Can you work these out from the model? Positions are in its coordinate system, mm. A direction names the side the tool comes from. Give positions to 0.01 mm unless a question says otherwise; leave off trailing zeros. Order: outer loops, then holes, each group sorted by start corner. A loop starts at its lowest first (then second) coordinate and runs counter-clockwise, first axis right, second up.
Item 1: I want a section at C-C, the plane x = 2.5. Write out the boundary of the cut face in (y, z), then the cut area to 3 significant figures.
Item 2: I want a section at A-A, the plane y = 0.2. Write out the boundary of the cut face in (x, z).
Item 3: If I drill on line 1 along Y through (x, z) = (1.25, 1); line 2 along Z through (x, y) = (-0.75, 0.3); line 3 along Z through (x, y) = (-1, 1), over which ranges is the centre line in solid material (lowest first)?
Item 4: If we mould it in two halves opening along Z, with no side actions, what happens to faces 6 (the flat face through (-1.73, 0.74, 4.57)), 7 (the flat face through (-2.957, 1, 5)), 8 (the flat face through (-0.35, 0.74, 0.97))? For each: +Z half, -Z half, draft (parallel to the pull), parting line (faces both ways), or undercut.
Item 5: I want a section at B-B, the plane z = 5. Write out the boundary of the cut face in (x, y), then the cut area to 3 significant figures.
Item 6: I want a section at D-D, the plane z = 2. Write out the boundary of the cut face in (x, y).
Item 7: Which directions (+Z, -Z, +X, -X, +Y, -Y) give clear straight access to the entire face, cutting with the end or side of a thin tool? Please do faces 1 (the flat face through (2.25, 1, -2)), 2 (the flat face through (-0.539, 1, 3)), 3 (the flat face through (-0.324, 1, -3)), 4 (the flat face through (-3.024, 1, 2)), 5 (the flat face through (-1.765, 0.74, 3.095)).
```python
from build123d import *

# Parameters (mm, degrees)
EXTRUDE_1_DEPTH   = 1.5
EXTRUDE_1_2_DEPTH = 1.5
EXTRUDE_1_3_DEPTH = 1.5
SKETCH_2_W        = 6.224573854
SKETCH_2_H        = 11.35798735
EXTRUDE_2_DEPTH   = 0.3


with BuildPart() as part:
    # Sketch 1 → Extrude 1 (new body)
    with BuildSketch(Plane(origin=(0, 0, 0), x_dir=(1, 0, 0), z_dir=(0, 1, 0))):
        Polygon((2.250249032, 2.455487133), (2.250249032, 0.954155558), (-3.02390068, -2.945886183), (-3.02390068, -1.444554608), align=None)
    extrude(amount=EXTRUDE_1_DEPTH)



with BuildPart() as body_2:
    # Sketch 1 → Extrude 1 2 (new body)
    with BuildSketch(Plane(origin=(0, 0, 0), x_dir=(1, 0, 0), z_dir=(0, 1, 0))):
        Polygon((2.093564175, 5.11615287), (2.093564175, 3.614821296), (-0.323874137, 1.827213654), (-0.323874137, 3.328545229), align=None)
    extrude(amount=EXTRUDE_1_2_DEPTH)


with BuildPart() as body_3:
    # Sketch 1 → Extrude 1 3 (new body)
    with BuildSketch(Plane(origin=(0, 0, 0), x_dir=(1, 0, 0), z_dir=(0, 1, 0))):
        Polygon((-0.539241249, -2.188970073), (-0.539241249, -3.690301647), (-2.956679561, -5.477909289), (-2.956679561, -3.976577714), align=None)
    extrude(amount=EXTRUDE_1_3_DEPTH)


with BuildPart() as part_1:
    add(part.part)

    add(body_2.part)  # Extrude 2 merges body 2

    add(body_3.part)  # Extrude 2 merges body 3
    # Sketch 2 → Extrude 2 (add)
    with BuildSketch(Plane(origin=(0, 1.5, 0), x_dir=(1, 0, 0), z_dir=(0, 1, 0))):
        with Locations((-0.374426275, -0.143679561)):
            Rectangle(SKETCH_2_W, SKETCH_2_H)
    extrude(amount=EXTRUDE_2_DEPTH)


solid = part_1.part
```
Results list:
1. outline: (1.5, -5.54) - (1.8, -5.54) - (1.8, 5.82) - (1.5, 5.82) - close
1. area: 3.41 mm2
2. outline: (-3.02, 1.44) - (2.25, -2.46) - (2.25, -0.95) - (-3.02, 2.95) - close; (-2.96, 3.98) - (-0.54, 2.19) - (-0.54, 3.69) - (-2.96, 5.48) - close; (-0.32, -3.33) - (2.09, -5.12) - (2.09, -3.61) - (-0.32, -1.83) - close
3. line 1: y = 1.5 to 1.8
3. line 2: z = -0.24 to 1.26, 2.34 to 3.85
3. line 3: z = -0.05 to 1.45, 2.53 to 4.03
4. face 6: +Z half
4. face 7: draft
4. face 8: undercut
5. outline: (-3.49, 1.5) - (-2.96, 1.5) - (-2.96, 0) - (-2.31, 0) - (-2.31, 1.5) - (2.74, 1.5) - (2.74, 1.8) - (-3.49, 1.8) - close
5. area: 2.84 mm2
6. outline: (-3.49, 1.5) - (-3.02, 1.5) - (-3.02, 0) - (-1.74, 0) - (-1.74, 1.5) - (2.74, 1.5) - (2.74, 1.8) - (-3.49, 1.8) - close
7. face 1: +Z, -Z, +X, -Y
7. face 2: +Z, +X, -Y
7. face 3: -Z, -X, -Y
7. face 4: +Z, -Z, -X, -Y
7. face 5: -Y
